from build123d import *

# Parameters (mm, degrees)
SALIENTE_EXTRUIR1_DEPTH = 2
SALIENTE_EXTRUIR2_DEPTH = 3.5
SALIENTE_EXTRUIR3_DEPTH = 5.5


with BuildPart() as part:
    # Croquis1 → Saliente-Extruir1 (new body)
    with BuildSketch(Plane.XY):
        Polygon((94.631182175, -5.210576854), (102.486249967, -9.756789114), (108.167092376, 0.058723162), (102.507485031, 9.885444115), (94.993770531, 5.545656204), (96.36344276, 2.872304936), (96.133929876, -2.614088967), align=None)
    extrude(amount=SALIENTE_EXTRUIR1_DEPTH)

    # Croquis2 → Saliente-Extruir2 (add)
    with BuildSketch(Plane(origin=(0, 0, 0), x_dir=(-1, 0, 0), z_dir=(0, 0, -1))):
        Polygon((-100.000000028, -1.2e-08), (-96.341228634, -6.200286222), (-94.631182175, -5.210576854), (-96.133929876, -2.614088967), (-96.36344276, 2.872304936), (-94.993770531, 5.545656204), (-96.346967159, 6.327238518), align=None)
        Polygon((-102.486249967, -9.756789114), (-100.841807638, -8.805048903), (-105.980454031, 0.073642516), (-100.862200724, 8.935157151), (-102.507485031, 9.885444115), (-108.167092376, 0.058723162), align=None)
    extrude(amount=SALIENTE_EXTRUIR2_DEPTH)

    # Croquis3 → Saliente-Extruir3 (add)
    with BuildSketch(Plane.XY.offset(2)):
        Polygon((94.631182175, -5.210576854), (96.133929876, -2.614088967), (96.36344276, 2.872304936), (94.993770531, 5.545656204), (96.248686318, 6.270473252), (99.795829711, 0.129107984), (96.184962548, -6.109845399), align=None)
    extrude(amount=SALIENTE_EXTRUIR3_DEPTH)


solid = part.part
Verification items for the finished model (mm, model axes). A direction names the side the tool comes from. Coordinates: 2 decimals unless noted, no trailing zeros. Write each loop counter-clockwise with the first axis right and the second up, starting at its lowest first coordinate (ties: lowest second). Pieces come first, ordered by that corner, then holes. Notation, with made-up numbers: (54, 36) -> (86, 36) arc R6 ccw to (86, 42) -> close; hole circle Ø3 at (82.5, 4). An arc over 180 degrees is marked (long way). One line per item, written item: value. Start each with the question number.
Q1. Cross-section at C-C on x = 105.5. Enter the section's corners in (y, z).
Q2. Cross-section at D-D on y = -4. Enter the section's corners in (x, z), and give its area (3 significant figures).
Q3. Mould release check, pull along X, two halves, no side actions. Record for faces 6 (the flat face through (98.196, -3.057, -1.726)), 7 (the flat face through (103.375, -4.428, -1.726)), 8 (the flat face through (105.287, -4.918, -0.788)), 9 (the flat face through (97, 0, -3.5)): pulls with the +X half, pulls with the -X half, needs draft (parallel to the pull), parting line crosses it, or undercut.
Q4. Cross-section at A-A on z = 5. Enter the section's corners in (x, y).
Q5. Access from +Z, -Z, +X, -X, +Y, -Y to the whole of each face (thin tool, end or side, straight path). Record for faces 1 (the flat face through (98.016, -2.947, 4.712)), 2 (the flat face through (95.69, 4.19, 1.92)), 3 (the flat face through (103.46, 4.44, -1.73)), 4 (the flat face through (98.148, 3.208, -1.726)), 5 (the flat face through (98, 3.24, 4.71)).
Q6. Cross-section at B-B on z = -0.25. Enter the section's corners in (x, y), and give its area (3 significant figures).
Q7. Go/stop test with flat-tipped pins: P1, Ø1, axis at x = 101.5, z = 3.5, coming from the -Y side; P2, Ø1, axis at y = -3, z = 0.5, coming from the +X side; P3, Ø3, axis at y = -3.5, z = 1.5, coming from the -X side; P4, Ø2, axis at y = -7, z = 0.5, coming from the -X side. Record where each tip stops, or that it passes through.
Q8. Thickness scan on L1, parallel to Z at x = 97.5, y = -5.5; L2, parallel to Z at x = 105.25, y = -2.5; L3, parallel to X at y = -6, z = -1.5. Record the ranges inside material, lowest first. Write a range as from..to.
Checked values:
1. outline: (-4.55, -3.5) -> (-0.76, -3.5) -> (-0.76, 0) -> (0.91, 0) -> (0.91, -3.5) -> (4.69, -3.5) -> (4.69, 2) -> (-4.55, 2) -> close
2. outline: (95.33, -3.5) -> (97.64, -3.5) -> (97.64, 0) -> (103.62, 0) -> (103.62, -3.5) -> (105.82, -3.5) -> (105.82, 2) -> (97.41, 2) -> (97.41, 7.5) -> (95.33, 7.5) -> close
2. area: 48.1 mm²
3. face 6: undercut
3. face 7: undercut
3. face 8: pulls with the +X half
3. face 9: needs draft
4. outline: (94.63, -5.21) -> (96.18, -6.11) -> (99.8, 0.13) -> (96.25, 6.27) -> (94.99, 5.55) -> (96.36, 2.87) -> (96.13, -2.61) -> close
5. face 1: +Z, +X, -Y
5. face 2: +Z, -Z, -X
5. face 3: -Z
5. face 4: -Z, +Y
5. face 5: +Z, +X, +Y
6. outline: (94.63, -5.21) -> (96.34, -6.2) -> (100, 0) -> (96.35, 6.33) -> (94.99, 5.55) -> (96.36, 2.87) -> (96.13, -2.61) -> close; (100.84, -8.81) -> (102.49, -9.76) -> (108.17, 0.06) -> (102.51, 9.89) -> (100.86, 8.94) -> (105.98, 0.07) -> close
6. area: 70.0 mm²
7. P1: passes through
7. P2: stops at x = 106.69
7. P3: stops at x = 94.75
7. P4: stops at x = 96
8. L1: z = 0..2
8. L2: z = -3.5..2
8. L3: x = 96..96.46, 102.47..104.66
